Here's how the part is built. I have some questions about the finished solid (model axes, mm). Face numbers are marked on the shaded views. A direction names the side the tool comes from. Coordinates: 2 decimals unless noted, no trailing zeros. Order: outer loops, then holes, each group sorted by start corner. A loop starts at its lowest first (then second) coordinate and runs counter-clockwise, first axis right, second up.
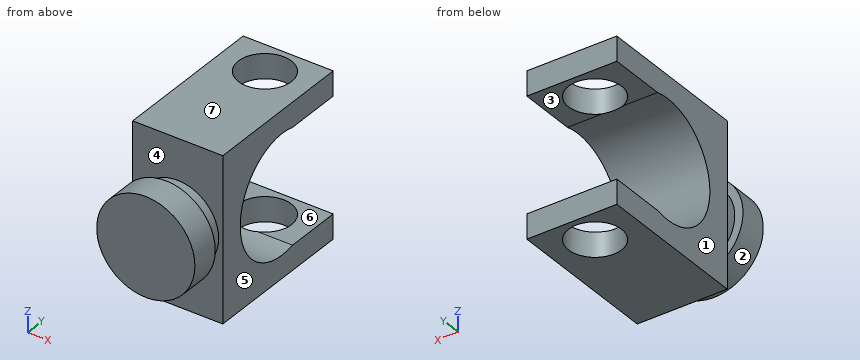
Autodesk Inventor part; units mm, degrees
ref_plane "YZ Plane" through (0, 0, 0) normal (1, 0, 0) x (0, 1, 0)
ref_plane "XZ Plane" through (0, 0, 0) normal (0, 1, 0) x (-1, 0, 0)
ref_plane "XY Plane" through (0, 0, 0) normal (0, 0, 1) x (1, 0, 0)
sketch "Sketch2" plane through (0, 0, 0) normal (0, 1, 0) x (-1, 0, 0)
  line L0 (0, 0) -> (0, -20)
  line L1 (0, -20) -> (11, -20)
  line L2 (11, -20) -> (11, 0)
  line L3 (11, 0) -> (0, 0)
  dimension "d3" = 11
  dimension "d35" = 20
extrude "Extrusion1" add sketch "Sketch2" along normal blind 15
sketch "Sketch3" plane through (-11, 0, 0) normal (0, 0, 1) x (1, 0, 0)
  line L0 (0, 0) -> (11, 0)
  line L1 (11, 0) -> (11, 15)
  line L2 (0, 15) -> (11, 15)
  line L3 (0, 0) -> (0, 15)
  line L4 (11, 15) -> (0, 15)
  circle A0 centre (5.5, 15) radius 3.25
  line L5 (0, 15) -> (0, 19)
  line L6 (0, 19) -> (11, 19)
  line L7 (11, 19) -> (11, 15)
  point P0 (8.75, 15)
  point P1 (2.25, 15)
  dimension "d33" = 6.5
  dimension "d34" = 4
extrude "Extrusion2" cut sketch "Sketch3" against normal blind 32.25 contours L2 A0 picked at (4.4481, 14.7407)
sketch "Sketch4" plane through (0, 0, 0) normal (1, 0, 0) x (0, 0, -1)
  line L0 (0, 0) -> (20, 0)
  line L1 (20, 0) -> (20, 15)
  line L2 (0, 15) -> (20, 15)
  line L3 (0, 0) -> (0, 15)
  line L4 (0, 15) -> (3, 15)
  line L5 (0, 15) -> (20, 15)
  line L6 (20, 15) -> (17, 15)
  line L7 (17, 15) -> (17, 12)
  line L8 (0, 11.75) -> (20, 11.75)
  line L9 (17, 12) -> (3, 12)
  line L10 (3, 12) -> (3, 15)
  line L11 (20, 0) -> (0, 0)
  line L12 (10, 0) -> (10, 3)
  arc A0 (3, 12) -> (17, 12) centre (10, 10.2222) ccw
  line L13 (3, 15) -> (3, 23.7535)
  line L14 (3, 23.7535) -> (17, 23.7535)
  line L15 (17, 23.7535) -> (17, 15)
  point P0 (17, 15)
  dimension "d11" = 3
  dimension "d12" = 3
  dimension "d36" = 3
  dimension "d37" = 3
extrude "Extrusion3" cut sketch "Sketch4" against normal blind 32.25 contours A0 L8 | A0 L9 L8 | L2 L7 L9 L10
sketch "Sketch7" plane through (0, 0, 0) normal (0, -1, 0) x (1, 0, 0)
  line L0 (0, -20) -> (-11, -20)
  line L1 (0, 0) -> (0, -20)
  line L2 (-11, 0) -> (0, 0)
  line L3 (-11, -20) -> (-11, 0)
  circle A0 centre (-5.5, -10) radius 5
  line L4 (-11, -3) -> (-11, 0)
  line L5 (-11, 0) -> (-11, -10)
  line L6 (-11, -17.2222) -> (-11, -2.7778)
  line L7 (-11, -10) -> (0, -10)
  line L8 (0, -2.7778) -> (0, -17.2222)
  line L9 (-8.75, 0) -> (-2.25, 0)
  line L10 (-5.5, 0) -> (-5.5, -10)
  point P0 (-11, -17)
  point P1 (0, -17)
  point P2 (0, -3)
  dimension "d22" = 10
  dimension "d38" = 10
extrude "Extrusion6" add sketch "Sketch7" along normal blind 2 contours L7 L10 A0 | A0 L7 | A0 L10 L7
sketch "Sketch8" plane through (-5.5, -2, -10) normal (0, -1, 0) x (1, 0, 0)
  circle A0 centre (0, 0) radius 6
  point P0 (5.5, 10)
  dimension "d25" = 12
extrude "Extrusion7" add sketch "Sketch8" along normal blind 3.5
extrude "Extrusion8" add sketch "Sketch3" against normal blind 20 contours L5 L6 L7 L2 A0
extrude "Extrusion9" cut sketch "Sketch4" against normal blind 26 contours L13 L14 L15 L2
Q1. If we section it at A-A on y = 16.25: Write out the boundary of the cut face in (x, z).
Q2. If we section it at B-B on z = -10: Write out the boundary of the cut face in (x, y).
Q3. We'd pull the mould along Z, two halves only. Please class the marked faces 5, 6 and 7: pulls with the +Z half, pulls with the -Z half, needs draft (parallel to the pull), parting line crosses it, or undercut.
Q4. Will these pins go through, and if not, where does the flat tip stop? pin 1 (5 mm diameter, centred on x = -4.5, z = -7.5, fed in from +Y); pin 2 (10 mm diameter, centred on y = 16.5, z = -3, fed in from -X); pin 3 (12 mm diameter, centred on y = 8, z = -3.5, fed in from +X).
Q5. If we section it at D-D on x = -5.75: Write out the boundary of the cut face in (y, z), then the cut area to 3 significant figures.
Q6. For the marked faces 1, 2, 3 and 4, which set-ups out of +Z, -Z, +X, -X, +Y, -Y let a thin tool reach every point of the face, with its end or its side?
Q7. If we section it at C-C on y = 10: Write out the boundary of the cut face in (x, z).
Q8. I need wall thicknesses on L1, parallel to Y at x = -5.5, z = -19.1; L2, parallel to X at y = 15, z = -1.3; L3, parallel to Z at x = -10, y = 17.25. Which ranges of each line are inside material? Lowest first, please.
Reply:
1. outline: (-11, -20) - (-8.5, -20) - (-8.5, -17) - (-11, -17) - close; (-11, -3) - (-8.5, -3) - (-8.5, 0) - (-11, 0) - close; (-2.5, -20) - (0, -20) - (0, -17) - (-2.5, -17) - close; (-2.5, -3) - (0, -3) - (0, 0) - (-2.5, 0) - close
2. outline: (-11.5, -5.5) - (0.5, -5.5) - (0.5, -2) - (-0.5, -2) - (-0.5, 0) - (0, 0) - (0, 3) - (-11, 3) - (-11, 0) - (-10.5, 0) - (-10.5, -2) - (-11.5, -2) - close
3. face 5: needs draft
3. face 6: undercut
3. face 7: pulls with the +Z half
4. pin 1: stops at y = 5.01
4. pin 2: stops at x = -11
4. pin 3: stops at x = 0
5. outline: (-5.5, -15.99) - (-2, -15.99) - (-2, -14.99) - (0, -14.99) - (0, -20) - (11.76, -20) - (11.76, -17.06) arc R7.22 cw (long way) to (11.76, -2.94) - (11.76, 0) - (0, 0) - (0, -5.01) - (-2, -5.01) - (-2, -4.01) - (-5.5, -4.01) - close; (18.24, -20) - (19, -20) - (19, -17) - (18.24, -17) - close; (18.24, -3) - (19, -3) - (19, 0) - (18.24, 0) - close
5. area: 198 mm2
6. face 1: +Z, -Z, -X, +Y
6. face 2: -Y
6. face 3: +X, -X, +Y
6. face 4: none
7. outline: (-11, -20) - (0, -20) - (0, -17.22) - (-11, -17.22) - close; (-11, -2.78) - (0, -2.78) - (0, 0) - (-11, 0) - close
8. L1: y = 0 to 11.75, 18.25 to 19
8. L2: x = -11 to -8.75, -2.25 to 0
8. L3: z = -20 to -17, -3 to 0
